Verification items for the finished model (mm, model axes). Round coordinates to 2 decimals unless told otherwise and drop trailing zeros. Loops run counter-clockwise (first coordinate to the right, second up) from the corner with the lowest first, then second, coordinate; pieces in that order, holes last. Notation, with made-up numbers: (-1.75, 67) -> (52.25, 67) arc R9 ccw to (52.25, 84) -> close; hole circle Ø4 at (40, 57). An arc over 180 degrees is marked (long way). Use CSV: the item, a comma, the result in double quotes. Start each with the question number.
```python
from build123d import *

# Parameters (mm, degrees)
SKETCH_1_R          = 90
SKETCH_1_R_2        = 2.1
SKETCH_1_R_3        = 20
EXTRUDE_1_DEPTH     = 4
SKETCH_2_R          = 1.6
CUT_EXTRUDE_1_DEPTH = 10


with BuildPart() as part:
    # 草图1 → 凸台-拉伸1 (new body)
    with BuildSketch(Plane.XY):
        Circle(SKETCH_1_R)
        with Locations((12.5, 80)):
            Circle(SKETCH_1_R_2, mode=Mode.SUBTRACT)
        with Locations((-12.5, 80)):
            Circle(SKETCH_1_R_2, mode=Mode.SUBTRACT)
        with Locations(Location((12.5, 60, 0), (0, 0, 180))):
            Circle(SKETCH_1_R_2, mode=Mode.SUBTRACT)
        with Locations(Location((-12.5, 60, 0), (0, 0, 180))):
            Circle(SKETCH_1_R_2, mode=Mode.SUBTRACT)
        Circle(SKETCH_1_R_3, mode=Mode.SUBTRACT)
        with Locations((75.532032303, -29.174682453)):
            Circle(SKETCH_1_R_2, mode=Mode.SUBTRACT)
        with Locations(Location((58.211524227, -19.174682453, 0), (0, 0, 180))):
            Circle(SKETCH_1_R_2, mode=Mode.SUBTRACT)
        with Locations(Location((45.711524227, -40.825317547, 0), (0, 0, 180))):
            Circle(SKETCH_1_R_2, mode=Mode.SUBTRACT)
        with Locations((63.032032303, -50.825317547)):
            Circle(SKETCH_1_R_2, mode=Mode.SUBTRACT)
        with Locations((-63.032032303, -50.825317547)):
            Circle(SKETCH_1_R_2, mode=Mode.SUBTRACT)
        with Locations(Location((-45.711524227, -40.825317547, 0), (0, 0, 180))):
            Circle(SKETCH_1_R_2, mode=Mode.SUBTRACT)
        with Locations(Location((-58.211524227, -19.174682453, 0), (0, 0, 180))):
            Circle(SKETCH_1_R_2, mode=Mode.SUBTRACT)
        with Locations((-75.532032303, -29.174682453)):
            Circle(SKETCH_1_R_2, mode=Mode.SUBTRACT)
    extrude(amount=EXTRUDE_1_DEPTH)

    # 草图2 → 切除-拉伸1 (cut)
    with BuildSketch(Plane.XY.offset(4)):
        with Locations((0, -70)):
            Circle(SKETCH_2_R)
        with Locations((-60.621778265, 35)):
            Circle(SKETCH_2_R)
        with Locations((60.621778265, 35)):
            Circle(SKETCH_2_R)
    extrude(amount=-CUT_EXTRUDE_1_DEPTH, mode=Mode.SUBTRACT)


solid = part.part
```
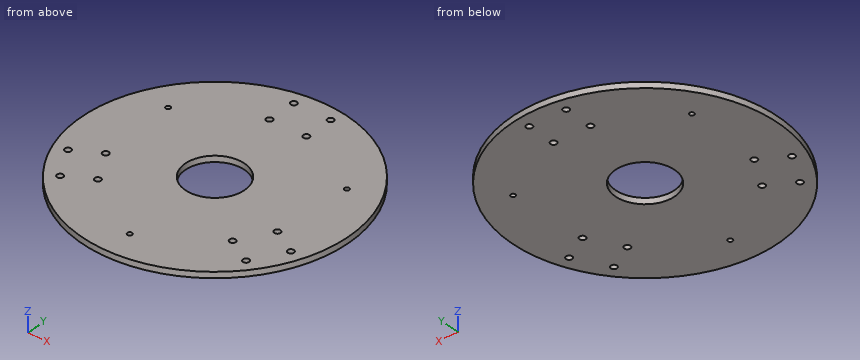
Q1. Thickness scan on L1, parallel to X at y = -18, z = 2.7; L2, parallel to X at y = -0.5, z = 0.6; L3, parallel to Y at x = 0, z = 2.45. Record the ranges inside material, lowest first. Write a range as from..to.
Q2. Cross-section at B-B (z = 2.55). State how many separate pieces and enclosed holes the cut face has, and give its area (3 significant figures).
Q3. Cross-section at D-D (y = 80). Record the boundary of the cut face in (x, z), and give its area (3 significant figures).
Q4. Cross-section at C-C (x = 12.5). Record the boundary of the cut face in (y, z), and give its area (3 significant figures).
Q5. Cross-section at A-A (y = 3.5). Record the boundary of the cut face in (x, z), and give its area (3 significant figures).
Q6. Depth check by flat-ended pin: pin 1 Ø1.5 at (y, z) = (32, 2.5) entering from +X; pin 2 Ø1.5 at (x, z) = (56.5, 1) entering from -Y; pin 3 Ø1 at (x, z) = (-38.5, 2.5) entering from -Y. Enter the tip coordinate at first touch or a pass-through.
Answer list:
1,L1,"x = -88.18..-59.95, -56.47..-8.72, 8.72..56.47, 59.95..88.18"
1,L2,"x = -90..-19.99, 19.99..90"
1,L3,"y = -90..-71.6, -68.4..-20, 20..90"
2,separate pieces,"1"
2,enclosed holes,"16"
2,area,"24,000 mm2"
3,outline,"(-41.23, 0) -> (-14.6, 0) -> (-14.6, 4) -> (-41.23, 4) -> close; (-10.4, 0) -> (10.4, 0) -> (10.4, 4) -> (-10.4, 4) -> close; (14.6, 0) -> (41.23, 0) -> (41.23, 4) -> (14.6, 4) -> close"
3,area,"296 mm2"
4,outline,"(-89.13, 0) -> (-15.61, 0) -> (-15.61, 4) -> (-89.13, 4) -> close; (15.61, 0) -> (57.9, 0) -> (57.9, 4) -> (15.61, 4) -> close; (62.1, 0) -> (77.9, 0) -> (77.9, 4) -> (62.1, 4) -> close; (82.1, 0) -> (89.13, 0) -> (89.13, 4) -> (82.1, 4) -> close"
4,area,"555 mm2"
5,outline,"(-89.93, 0) -> (-19.69, 0) -> (-19.69, 4) -> (-89.93, 4) -> close; (19.69, 0) -> (89.93, 0) -> (89.93, 4) -> (19.69, 4) -> close"
5,area,"562 mm2"
6,pin 1,"stops at x = 84.4"
6,pin 2,"stops at y = -70.65"
6,pin 3,"stops at y = -81.58"
